Design review of the part shown in the three views and the two pictorial views. Dimensions are in mm from the part's minimum x, y and z. A direction names the side the tool comes from. Coordinates: 2 decimals unless noted, no trailing zeros. Loops run counter-clockwise (first coordinate to the right, second up) from the corner with the lowest first, then second, coordinate; pieces in that order, holes last. Notation, with made-up numbers: (32, 0) -> (72, 0) arc R18 ccw to (72, 25) -> close; hole circle Ø4 at (24.5, 88.25). An arc over 180 degrees is marked (long way). Answer in a Markdown table with one row per item.
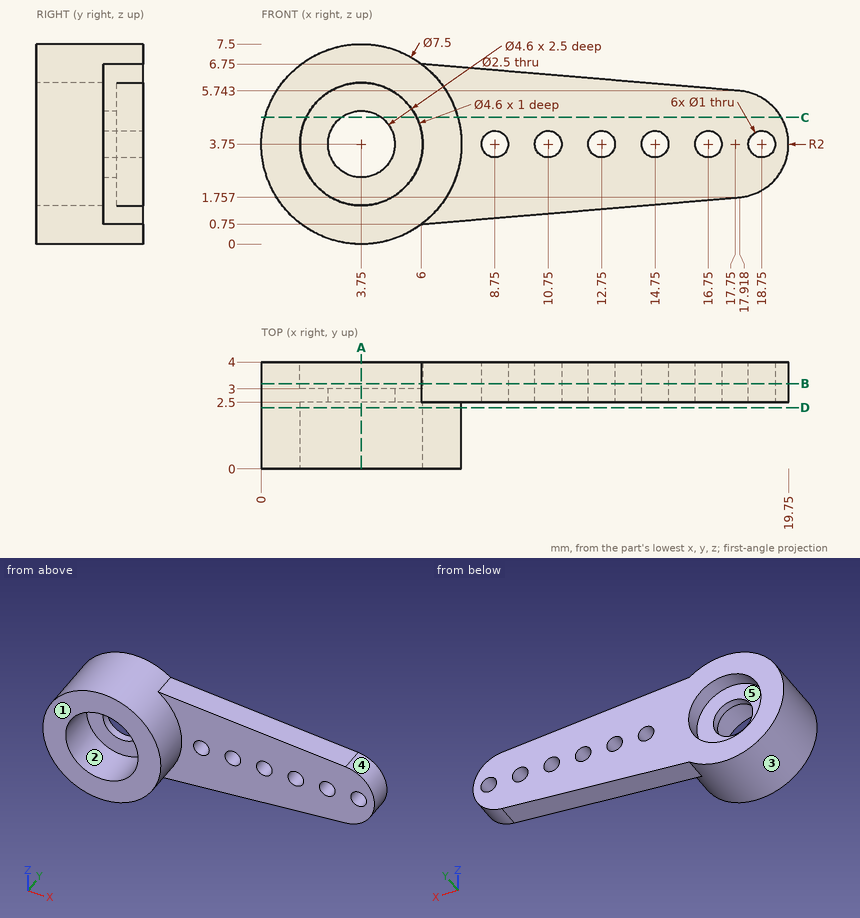
(1) Take a section at D-D on y = 2.3. Give the boundary of the cut face in (x, z).
Evaluation:
| item | result |
|---|---|
| outline | circle Ø7.5 at (3.75, 3.75); hole circle Ø4.6 at (3.75, 3.75) |
(2) For pin 1 (1.5 mm diameter, centred on y = 3, z = 5, fed in from -X); pin 2 (3.5 mm diameter, centred on x = 3.5, z = 5, fed in from -Y); pin 3 (1.4 mm diameter, centred on x = 3.5, z = 4.5, fed in from +Y), all flat-tipped, find the tip position at first contact; note any pin that passes through.
Evaluation:
| item | result |
|---|---|
| pin 1 | stops at x = 0.03 |
| pin 2 | stops at y = 0 |
| pin 3 | stops at y = 3 |
(3) Take a section at B-B on y = 3.2. Give the boundary of the cut face in (x, z).
Evaluation:
| item | result |
|---|---|
| outline | (6, 0.75) -> (17.92, 1.76) arc R2 ccw to (17.92, 5.74) -> (6, 6.75) arc R3.75 ccw (long way) to start; hole circle Ø4.6 at (3.75, 3.75); hole circle Ø1 at (8.75, 3.75); hole circle Ø1 at (10.75, 3.75); hole circle Ø1 at (12.75, 3.75); hole circle Ø1 at (14.75, 3.75); hole circle Ø1 at (16.75, 3.75); hole circle Ø1 at (18.75, 3.75) |
(4) To check wall thickness, follow probe 1 along Z at (x, y) = (3.75, 3.75); probe 2 along Z at (x, y) = (12.75, 3.25); probe 3 along Y at (x, z) = (12, 5.25). State the ranges of each line that lie inside material, in increasing order.
Evaluation:
| item | result |
|---|---|
| probe 1 | z = 0 to 1.45, 6.05 to 7.5 |
| probe 2 | z = 1.32 to 3.25, 4.25 to 6.18 |
| probe 3 | y = 2.5 to 4 |
(5) Draft analysis for pull direction X (two halves, no side actions). For the marked faces 3, 4 and 5, state which applies: pulls with the +X half, pulls with the -X half, needs draft (parallel to the pull), parting line crosses it, or undercut.
Evaluation:
| item | result |
|---|---|
| face 3 | parting line crosses it |
| face 4 | pulls with the +X half |
| face 5 | undercut |
(6) Take a section at A-A on x = 3.75. Give the boundary of the cut face in (y, z).
Evaluation:
| item | result |
|---|---|
| outline | (0, 0) -> (4, 0) -> (4, 1.45) -> (3, 1.45) -> (3, 2.5) -> (2.5, 2.5) -> (2.5, 1.45) -> (0, 1.45) -> close; (0, 6.05) -> (2.5, 6.05) -> (2.5, 5) -> (3, 5) -> (3, 6.05) -> (4, 6.05) -> (4, 7.5) -> (0, 7.5) -> close |
(7) Tool access review of the marked faces 1 and 2: name each direction out of +Z, -Z, +X, -X, +Y, -Y from which nothing blocks a thin tool from reaching the whole face with its end or side.
Evaluation:
| item | result |
|---|---|
| face 1 | +Z, -Z, +X, -X, -Y |
| face 2 | -Y |
(8) Take a section at C-C on z = 4.75. Give the boundary of the cut face in (x, y) (1 decimal).
Evaluation:
| item | result |
|---|---|
| outline | (0.1, 0) -> (1.7, 0) -> (1.7, 2.5) -> (3, 2.5) -> (3, 3) -> (1.7, 3) -> (1.7, 4) -> (0.1, 4) -> close; (4.5, 2.5) -> (5.8, 2.5) -> (5.8, 0) -> (7.4, 0) -> (7.4, 2.5) -> (19.5, 2.5) -> (19.5, 4) -> (5.8, 4) -> (5.8, 3) -> (4.5, 3) -> close |
